from build123d import *

# Parameters (mm, degrees)
EXTRUDE_1_DEPTH      = 2
EXTRUDE_2_DEPTH      = 10
EXTRUDE_2_DEPTH_BACK = 2
SKETCH_2_W           = 2
SKETCH_2_H           = 20
SKETCH_2_W_2         = 20
SKETCH_2_H_2         = 2
SKETCH_3_R           = 1.65
CUT_EXTRUDE_1_DEPTH  = 12
SKETCH_4_R           = 1.65
CUT_EXTRUDE_2_DEPTH  = 12
FILLET_1_R           = 2


with BuildPart() as part:
    # 草图1 → 凸台-拉伸1 (new body)
    with BuildSketch(Plane.XY):
        with BuildLine():
            Line((4, 0), (109.5, 0))
            ThreePointArc((109.5, 0), (112.328427125, 1.171572875), (113.5, 4))
            Line((113.5, 4), (113.5, 76.5))
            ThreePointArc((113.5, 76.5), (112.328427125, 79.328427125), (109.5, 80.5))
            Line((109.5, 80.5), (4, 80.5))
            ThreePointArc((4, 80.5), (1.171572875, 79.328427125), (0, 76.5))
            Line((0, 76.5), (0, 4))
            ThreePointArc((0, 4), (1.171572875, 1.171572875), (4, 0))
        make_face()
    extrude(amount=EXTRUDE_1_DEPTH)

    # 草图2 → 凸台-拉伸2 (add, two sides: drawn at the far end of the back side and taken through both)
    with BuildSketch(Plane.XY.offset(2).offset(-EXTRUDE_2_DEPTH_BACK)):
        with Locations((114.5, 40)):
            Rectangle(SKETCH_2_W, SKETCH_2_H)
        with Locations((30, -1)):
            Rectangle(SKETCH_2_W_2, SKETCH_2_H_2)
        with Locations((83.5, -1)):
            Rectangle(SKETCH_2_W_2, SKETCH_2_H_2)
    extrude(amount=EXTRUDE_2_DEPTH + EXTRUDE_2_DEPTH_BACK)

    # 草图3 → 切除-拉伸1 (cut)
    with BuildSketch(Plane(origin=(115.5, 0, 0), x_dir=(0, 0, -1), z_dir=(1, 0, 0))):
        with Locations((-7, 40)):
            Circle(SKETCH_3_R)
    extrude(amount=-CUT_EXTRUDE_1_DEPTH, mode=Mode.SUBTRACT)

    # 草图4 → 切除-拉伸2 (cut)
    with BuildSketch(Plane(origin=(0, -2, 0), x_dir=(-1, 0, 0), z_dir=(0, -1, 0))):
        with Locations(Location((-83.5, -7, 0), (0, 0, 180))):
            Circle(SKETCH_4_R)
        with Locations(Location((-30, -7, 0), (0, 0, 180))):
            Circle(SKETCH_4_R)
    extrude(amount=-CUT_EXTRUDE_2_DEPTH, mode=Mode.SUBTRACT)

    # 圆角1
    fillet_1_edges = [part.edges().sort_by_distance(p)[0] for p in [
        (113.5, 50, 1),
        (113.5, 30, 1),
        (40, 0, 1),
        (20, 0, 1),
        (73.5, 0, 1),
        (93.5, 0, 1),
    ]]
    fillet(fillet_1_edges, radius=FILLET_1_R - 0.0001)  # a hair under: the kernel refuses the full size


solid = part.part
Build history of the part. All positions in model axes, mm. A direction names the side the tool comes from. Give positions to 0.01 mm unless a question says otherwise; leave off trailing zeros. Order: outer loops, then holes, each group sorted by start corner. A loop starts at its lowest first (then second) coordinate and runs counter-clockwise, first axis right, second up. Notation, with made-up numbers: M 20.25,39.25 L 64.25,39.25 A19 cw 64.25,60.25 Z; hole C 52,26 d10. An arc over 180 degrees is marked long. Use one line per item in the form item = value.
Q1. Slice it at D-D, the plane x = 75.5. Write the cut outline in (y, z), and give its area (3 significant figures).
Conclusion:
outline = M -2,0 L 80.5,0 L 80.5,2 L 0,2 L 0,12 L -2,12 Z
area = 185 mm2
Q2. Pull direction X, two halves, no side cores. Call faces 3 (the cylindrical face through (28.69, -1.01, 6)), 4 (the flat face through (113.5, 38, 7)), 5 (the flat face through (28, 0, 7)): released by +X, released by -X, zero draft, split by the parting line, or undercut.
Conclusion:
face_3 = undercut
face_4 = released by -X
face_5 = zero draft
Q3. Slice it at C-C, the plane z = 7. Write the cut outline in (x, y).
Conclusion:
outline = M 20,-2 L 28.35,-2 L 28.35,0 L 20,0 Z; M 31.65,-2 L 40,-2 L 40,0 L 31.65,0 Z; M 73.5,-2 L 81.85,-2 L 81.85,0 L 73.5,0 Z; M 85.15,-2 L 93.5,-2 L 93.5,0 L 85.15,0 Z; M 113.5,30 L 115.5,30 L 115.5,38.35 L 113.5,38.35 Z; M 113.5,41.65 L 115.5,41.65 L 115.5,50 L 113.5,50 Z
Q4. Slice it at A-A, the plane x = 30. Write the cut outline in (y, z).
Conclusion:
outline = M -2,0 L 80.5,0 L 80.5,2 L 0,2 L 0,5.35 L -2,5.35 Z; M -2,8.65 L 0,8.65 L 0,12 L -2,12 Z
Q5. Slice it at B-B, the plane y = 40. Write the cut outline in (x, z), and give its area (3 significant figures).
Conclusion:
outline = M 0,0 L 115.5,0 L 115.5,5.35 L 113.5,5.35 L 113.5,2 L 0,2 Z; M 113.5,8.65 L 115.5,8.65 L 115.5,12 L 113.5,12 Z
area = 244 mm2
Q6. Pin check, flat tips, straight feed: P1, Ø2, axis at x = 29, y = 21, coming from the -Z side; P2, Ø1, axis at y = 26, z = 3, coming from the +X side; P3, Ø3, axis at y = 48, z = 7.5, coming from the -X side; P4, Ø0.6, axis at y = -1, z = 8, coming from the -X side. Stop position of each tip, or through.
Conclusion:
P1 = 0
P2 = through
P3 = 113.5
P4 = 20
Q7. Wall check: probe 1 along Z at (x, y) = (30, -0.4); probe 2 along X at (y, z) = (45, 9); probe 3 along Y at (x, z) = (115.15, 7). Give the ranges that are in metal, low to high.
Conclusion:
probe_1 = 0 to 5.35, 8.65 to 12
probe_2 = 113.5 to 115.5
probe_3 = 30 to 38.35, 41.65 to 50
Q8. Which spindle directions (+Z, -Z, +X, -X, +Y, -Y) get a long thin tool onto all of the face, cutting with end or side? Do faces 1 (the cylindrical face through (1.141, 1.203, 0.986)), 2 (the flat face through (86, 0, 7)). Say none if no direction does.
Conclusion:
face_1 = +Z, -Z, -X, -Y
face_2 = +Z, +X, -X, +Y
